Part print with two shaded views. Sizes in mm from the minimum x, y, z corner. Coordinates: 2 decimals unless noted, no trailing zeros. Write each loop counter-clockwise with the first axis right and the second up, starting at its lowest first coordinate (ties: lowest second). Pieces come first, ordered by that corner, then holes.
Q1. Pin check, flat tip, straight feed: P1, Ø1.5, axis at y = 21, z = 3.5, coming from the -X side. Stop position of the tip, or through.
Q2. Band-saw the part on B-B, the plane z = 1.5. Write the cut outline in (x, y), plus the area to 3 significant figures.
Q3. Drill centre lines: probe 1 along X at (y, z) = (29, 4.5); probe 2 along X at (y, z) = (13, 2). Where is each one in solid material? Low to high.
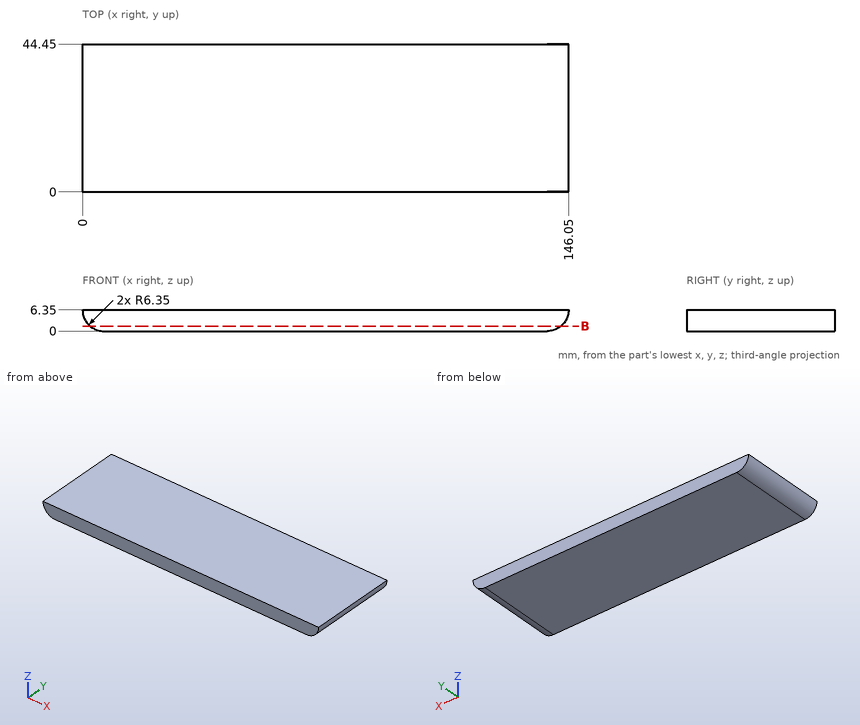
Answer sheet:
1. P1: stops at x = 0.36
2. outline: (2.25, 0) - (143.8, 0) - (143.8, 44.45) - (2.25, 44.45) - close
2. area: 6,290 mm2
3. probe 1: x = 0.28 to 145.77
3. probe 2: x = 1.72 to 144.33
